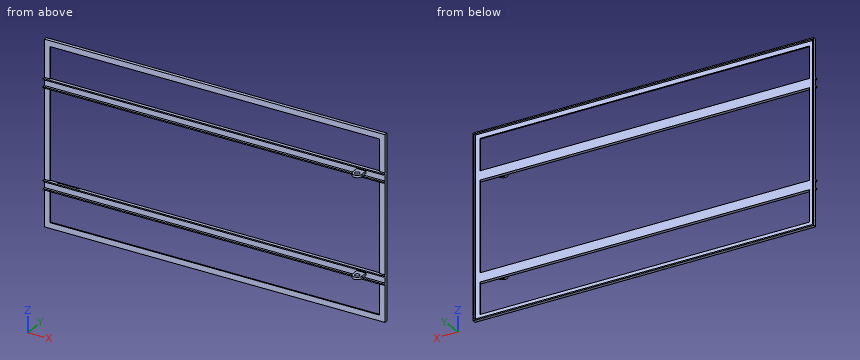
```python
from build123d import *

# Parameters (mm, degrees)
SKETCH2_W                 = 1510
SKETCH2_H                 = 810
SKETCH2_W_2               = 1500
SKETCH2_H_2               = 800
BOSS_EXTRUDE1_DEPTH       = 10
SKETCH3_W                 = 1510
SKETCH3_H                 = 810
SKETCH3_W_2               = 1460
SKETCH3_H_2               = 140
SKETCH3_W_3               = 30
SKETCH3_H_3               = 400
SKETCH3_W_4               = 1200
BOSS_EXTRUDE2_DEPTH       = 5
SKETCH5_W                 = 1510
SKETCH5_H                 = 5
BOSS_EXTRUDE3_DEPTH       = 10
LPATTERN1_COUNT           = 2
LPATTERN1_PITCH           = 35
LPATTERN2_COUNT           = 2
LPATTERN2_PITCH           = 440
LPATTERN2_COPY_1_SKETCH_W = 1510
LPATTERN2_COPY_1_SKETCH_H = 5
LPATTERN2_COPY_1_DEPTH    = 10
SKETCH6_R                 = 10
BOSS_EXTRUDE4_DEPTH       = 5
LPATTERN3_COUNT           = 2
LPATTERN3_PITCH           = 440
SKETCH7_W                 = 100
SKETCH7_H                 = 399.729040111
SKETCH7_H_2               = 400
CUT_EXTRUDE5_DEPTH        = 10


with BuildPart() as part:
    # Sketch2 → Boss-Extrude1 (new body)
    with BuildSketch(Plane(origin=(0, 0, 0), x_dir=(1, 0, 0), z_dir=(0, 1, 0))):
        Rectangle(SKETCH2_W, SKETCH2_H)
        Rectangle(SKETCH2_W_2, SKETCH2_H_2, mode=Mode.SUBTRACT)
    extrude(amount=BOSS_EXTRUDE1_DEPTH)

    # Sketch3 → Boss-Extrude2 (add)
    with BuildSketch(Plane(origin=(0, 0, 0), x_dir=(1, 0, 0), z_dir=(0, 1, 0))):
        Rectangle(SKETCH3_W, SKETCH3_H)
        with Locations((0, -310)):
            Rectangle(SKETCH3_W_2, SKETCH3_H_2, mode=Mode.SUBTRACT)
        with Locations((0, 310)):
            Rectangle(SKETCH3_W_2, SKETCH3_H_2, mode=Mode.SUBTRACT)
        with Locations((-715, 0)):
            Rectangle(SKETCH3_W_3, SKETCH3_H_3, mode=Mode.SUBTRACT)
        with Locations((715, 0)):
            Rectangle(SKETCH3_W_3, SKETCH3_H_3, mode=Mode.SUBTRACT)
        Rectangle(SKETCH3_W_4, SKETCH3_H_3, mode=Mode.SUBTRACT)
    extrude(amount=-BOSS_EXTRUDE2_DEPTH)

    # Sketch5 → Boss-Extrude3 (add)
    with BuildSketch(Plane.XZ.offset(5)):
        with Locations((0, 237.5)):
            Rectangle(SKETCH5_W, SKETCH5_H)
    boss_extrude3 = extrude(amount=BOSS_EXTRUDE3_DEPTH)

    # LPattern1: Boss-Extrude3 ×2
    with Locations(*[(0, 0, -i * LPATTERN1_PITCH) for i in range(1, LPATTERN1_COUNT)]):
        add(boss_extrude3)

    # LPattern2: Boss-Extrude3 ×2
    with Locations(*[(0, 0, -i * LPATTERN2_PITCH) for i in range(1, LPATTERN2_COUNT)]):
        add(boss_extrude3)

    # LPattern2 copy 1 sketch → LPattern2 copy 1 (add)
    with BuildSketch(Plane(origin=(0, -5, -475), x_dir=(1, 0, 0), z_dir=(0, -1, 0))):
        with Locations((0, 237.5)):
            Rectangle(LPATTERN2_COPY_1_SKETCH_W, LPATTERN2_COPY_1_SKETCH_H)
    extrude(amount=LPATTERN2_COPY_1_DEPTH)

    # Sketch6 → Boss-Extrude4 (add, symmetric)
    with BuildSketch(Plane.XY.offset(220)):
        with BuildLine():
            Line((630, -5), (630, -35))
            ThreePointArc((630, -35), (650, -55), (670, -35))
            Line((670, -35), (670, -5))
            Line((670, -5), (630, -5))
        make_face()
        with Locations((650, -35)):
            Circle(SKETCH6_R, mode=Mode.SUBTRACT)
    boss_extrude4 = extrude(amount=BOSS_EXTRUDE4_DEPTH, both=True)

    # LPattern3: Boss-Extrude4 ×2
    with Locations(*[(0, 0, -i * LPATTERN3_PITCH) for i in range(1, LPATTERN3_COUNT)]):
        add(boss_extrude4)

    # Sketch7 → Cut-Extrude5 (cut)
    with BuildSketch(Plane.XZ.offset(5)):
        with Locations((-650, 0.135479944)):
            Rectangle(SKETCH7_W, SKETCH7_H)
        with Locations((650, 0)):
            Rectangle(SKETCH7_W, SKETCH7_H_2)
    extrude(amount=-CUT_EXTRUDE5_DEPTH, mode=Mode.SUBTRACT)


solid = part.part
```
Part model, mm, in its own coordinate system. Give positions to 0.01 mm unless a question says otherwise; leave off trailing zeros. Loops run counter-clockwise (first coordinate to the right, second up) from the corner with the lowest first, then second, coordinate; pieces in that order, holes last. Notation, with made-up numbers: M 67.5,1.25 L 102.5,1.25 A24 cw 102.5,12.25 Z; hole C -37,75 d1. An arc over 180 degrees is marked long. Return JSON: item names as keys, results as strings.
1) Saw through at B-B, the plane z = -172. List the corners of the cut face in (x, y).
Calculated:
{"outline": "M -755,-5 L -730,-5 L -730,0 L -750,0 L -750,10 L -755,10 Z; M 730,-5 L 755,-5 L 755,10 L 750,10 L 750,0 L 730,0 Z"}
2) Flat gauge pins, fed straight in: pin 1 Ø3 at (x, y) = (-565, -11) entering from +Z; pin 2 Ø20 at (x, y) = (652.5, -35.5) entering from -Z; pin 3 Ø4.5 at (x, y) = (65.5, -10) entering from -Z; pin 4 Ø8 at (x, y) = (31, -21) entering from +Z. Where does each tip first touch, or does it go through?
Calculated:
{"pin 1": "stops at z = 240", "pin 2": "stops at z = -225", "pin 3": "stops at z = -240", "pin 4": "passes through"}
3) Drill centre lines: line 1 (Z direction, x = -71, y = -13); line 2 (Y direction, x = 650, z = 221.5); line 3 (X direction, y = 3.5, z = -275). Where is each one in solid material? Low to high.
Calculated:
{"line 1": "z = -240 to -235, -205 to -200, 200 to 205, 235 to 240", "line 2": "y = -55 to -45, -25 to 0", "line 3": "x = -755 to -750, 750 to 755"}
4) Saw through at A-A, the plane x = 103. List the corners of the cut face in (y, z), then the cut area to 3 significant figures.
Calculated:
{"outline": "M -15,-240 L 0,-240 L 0,-200 L -15,-200 L -15,-205 L -5,-205 L -5,-235 L -15,-235 Z; M -15,200 L 0,200 L 0,240 L -15,240 L -15,235 L -5,235 L -5,205 L -15,205 Z; M -5,-405 L 10,-405 L 10,-400 L 0,-400 L 0,-380 L -5,-380 Z; M -5,380 L 0,380 L 0,400 L 10,400 L 10,405 L -5,405 Z", "area": "950 mm2"}
